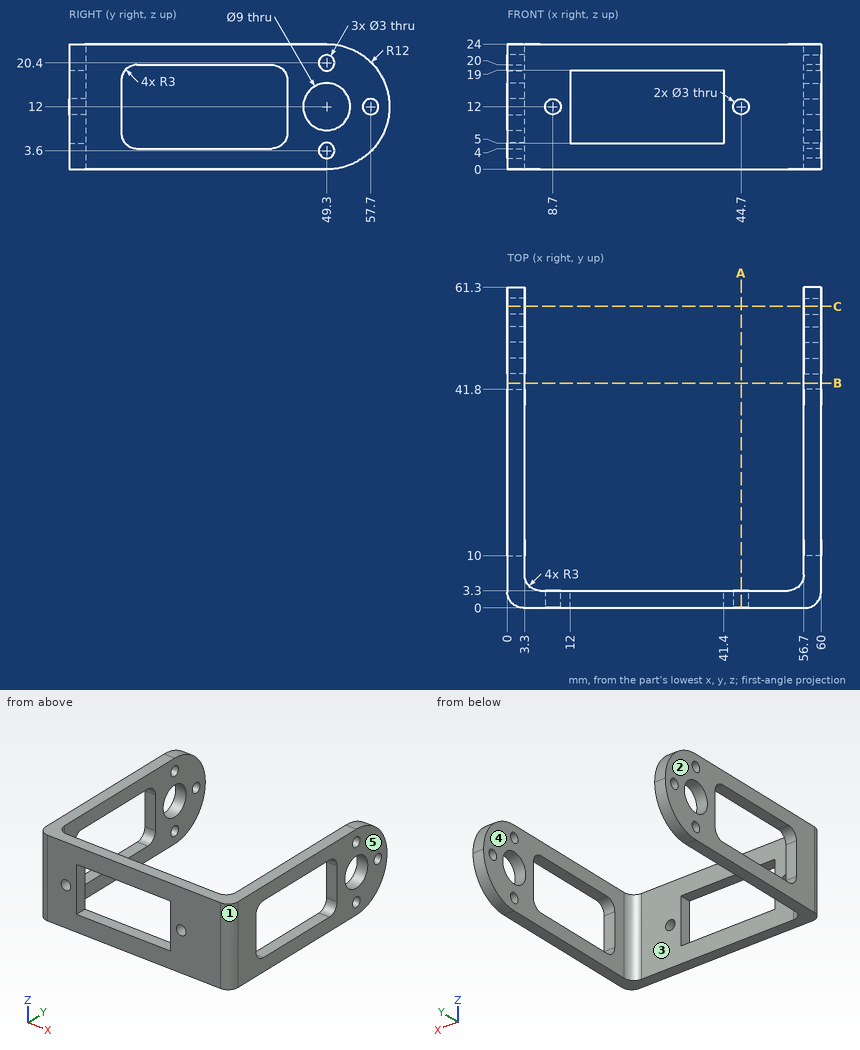
Job drawing, mm, ordinate dimensions from the low corner. One solid piece. A direction names the side the tool comes from. Round coordinates to 2 decimals unless told otherwise and drop trailing zeros. Write each loop counter-clockwise with the first axis right and the second up, starting at its lowest first coordinate (ties: lowest second). Pieces come first, ordered by that corner, then holes.
1) Mould opens along X. For the marked faces 1, 2 and 3 say: +X half, -X half, draft (parallel to the pull), parting line (faces both ways), or undercut.
2) Band-saw the part on B-B, the plane y = 43. List the corners of the cut face in (x, z).
3) 3-axis set-ups, long thin cutter, end or side, ignore diameter. For the marked faces 4 and 5: which of +Z, -Z, +X, -X, +Y, -Y reach the whole face in a straight line?
4) Drill centre lines: probe 1 along X at (y, z) = (52, 5.5); probe 2 along X at (y, z) = (1.1, 12); probe 3 along Y at (x, z) = (50.5, 9.5). Where is each one in solid material? Low to high.
5) Pin check, flat tips, straight feed: pin 1 (2 mm diameter, centred on x = 8, z = 7, fed in from +Y); pin 2 (1 mm diameter, centred on y = 1, z = 15.5, fed in from -X); pin 3 (1.5 mm diameter, centred on y = 38, z = 5, fed in from +X). Stop position of each tip, or through.
6) Band-saw the part on A-A, the plane x = 44.7. List the corners of the cut face in (y, z).
7) Band-saw the part on C-C, the plane y = 57.7. List the corners of the cut face in (x, z), and give its area (3 significant figures).
Ans:
1. face 1: +X half
1. face 2: -X half
1. face 3: undercut
2. outline: (0, 0) - (3.3, 0) - (3.3, 24) - (0, 24) - close; (56.7, 0) - (60, 0) - (60, 24) - (56.7, 24) - close
3. face 4: +Z, -Z, +Y
3. face 5: +Z, -Z, +X, +Y, -Y
4. probe 1: x = 0 to 3.3, 56.7 to 60
4. probe 2: x = 0.68 to 7.2, 10.2 to 12, 41.4 to 43.2, 46.2 to 59.32
4. probe 3: y = 0 to 3.3
5. pin 1: stops at y = 3.3
5. pin 2: stops at x = 0.4
5. pin 3: passes through
6. outline: (0, 0) - (3.3, 0) - (3.3, 10.5) - (0, 10.5) - close; (0, 13.5) - (3.3, 13.5) - (3.3, 24) - (0, 24) - close
7. outline: (0, 3.43) - (3.3, 3.43) - (3.3, 10.5) - (0, 10.5) - close; (0, 13.5) - (3.3, 13.5) - (3.3, 20.57) - (0, 20.57) - close; (56.7, 3.43) - (60, 3.43) - (60, 10.5) - (56.7, 10.5) - close; (56.7, 13.5) - (60, 13.5) - (60, 20.57) - (56.7, 20.57) - close
7. area: 93.3 mm2
